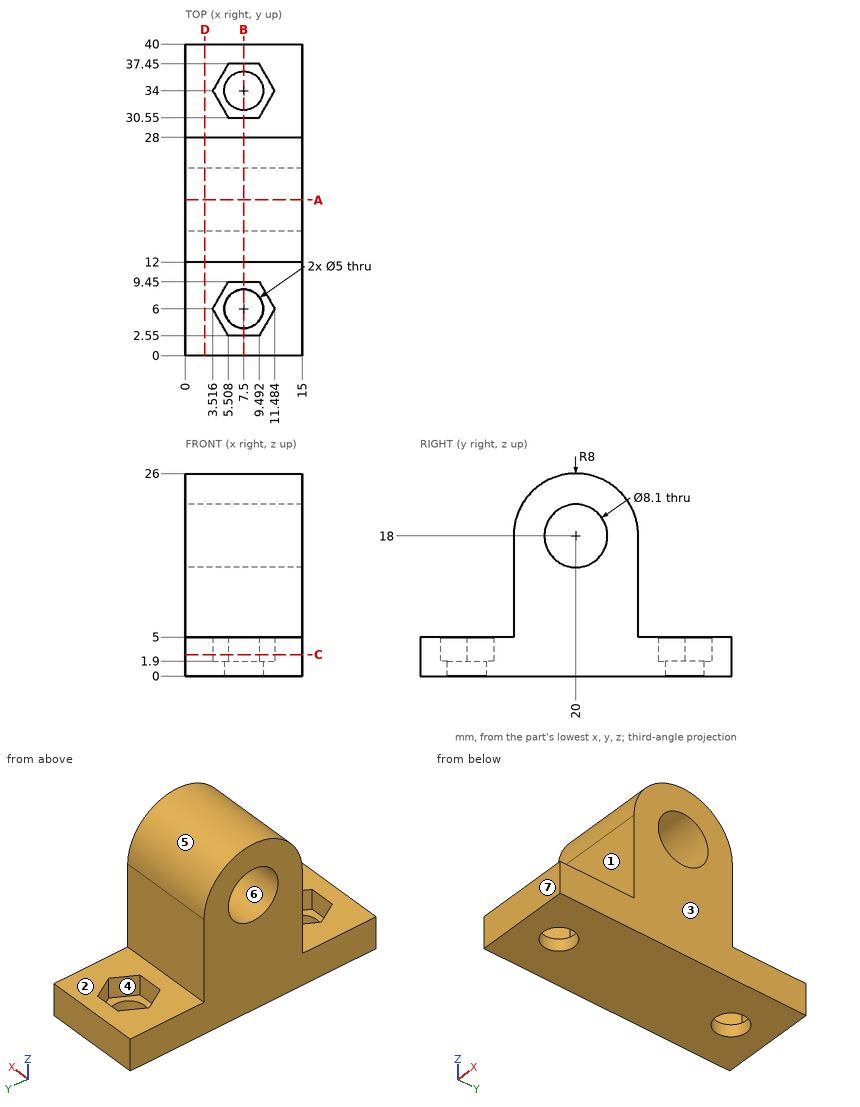
Geometry check sheet. Reference: drawing and pictorial views, mm from the part's lowest x, y, z. A direction names the side the tool comes from. Give positions to 0.01 mm unless a question says otherwise; leave off trailing zeros. Order: outer loops, then holes, each group sorted by start corner. A loop starts at its lowest first (then second) coordinate and runs counter-clockwise, first axis right, second up. Notation, with made-up numbers: (84, 18) -> (143, 18) arc R26 ccw to (143, 45) -> close; hole circle Ø2 at (9, 17.25). An arc over 180 degrees is marked (long way). Use CSV: the item, a comma, the result in double quotes. Start each with the question number.
1) Sectioned sample at A-A, the plane y = 20. Record the boundary of the cut face in (x, z).
2) Sectioned sample at C-C, the plane z = 2.75. Record the boundary of the cut face in (x, y).
3) Go/stop test with flat-tipped pins: P1, Ø2, axis at x = 7, y = 33.5, coming from the +Z side; P2, Ø5.5, axis at x = 7, y = 7, coming from the +Z side; P3, Ø4, axis at x = 11, z = 9, coming from the +Y side; P4, Ø4, axis at x = 4.5, z = 11.5, coming from the -Y side. Record where each tip stops, or that it passes through.
4) Sectioned sample at B-B, the plane x = 7.5. Record the boundary of the cut face in (y, z), plus the area to 3 significant figures.
5) Set-up check for the marked faces 1, 2 and 3: record each of +Z, -Z, +X, -X, +Y, -Y from which the full face is reachable in a straight line by a thin tool's end or side.
6) Material ranges on line 1 (X direction, y = 6, z = 0.8); line 2 (Z direction, x = 9.75, y = 20); line 3 (Z direction, x = 5, y = 18) (1 decimal), recorded low to high. Write a range as from..to.
7) Sectioned sample at D-D, the plane x = 2.5. Record the boundary of the cut face in (y, z), plus the area to 3 significant figures.
8) Mould release check, pull along Y, two halves, no side actions. Record for the marked faces 4, 5, 6 and 7: released by +Y, released by -Y, zero draft, split by the parting line, or undercut.
Recorded:
1,outline,"(0, 0) -> (15, 0) -> (15, 13.95) -> (0, 13.95) -> close; (0, 22.05) -> (15, 22.05) -> (15, 26) -> (0, 26) -> close"
2,outline,"(0, 0) -> (15, 0) -> (15, 40) -> (0, 40) -> close; hole (3.52, 6) -> (5.51, 2.55) -> (9.49, 2.55) -> (11.48, 6) -> (9.49, 9.45) -> (5.51, 9.45) -> close; hole (3.52, 34) -> (5.51, 30.55) -> (9.49, 30.55) -> (11.48, 34) -> (9.49, 37.45) -> (5.51, 37.45) -> close"
3,P1,"through"
3,P2,"z = 5"
3,P3,"y = 28"
3,P4,"y = 12"
4,outline,"(0, 0) -> (3.5, 0) -> (3.5, 1.9) -> (2.55, 1.9) -> (2.55, 5) -> (0, 5) -> close; (8.5, 0) -> (31.5, 0) -> (31.5, 1.9) -> (30.55, 1.9) -> (30.55, 5) -> (28, 5) -> (28, 18) arc R8 ccw to (12, 18) -> (12, 5) -> (9.45, 5) -> (9.45, 1.9) -> (8.5, 1.9) -> close; (36.5, 0) -> (40, 0) -> (40, 5) -> (37.45, 5) -> (37.45, 1.9) -> (36.5, 1.9) -> close; hole circle Ø8.1 at (20, 18)"
4,area,"395 mm2"
5,face 1,"+Z, +X, -X, -Y"
5,face 2,"+Z, +X, -X, +Y"
5,face 3,"+Z, -Z, +X, +Y, -Y"
6,line 1,"0..5, 10..15"
6,line 2,"0..13.95, 22.05..26"
6,line 3,"0..14.5, 21.5..25.7"
7,outline,"(0, 0) -> (40, 0) -> (40, 5) -> (28, 5) -> (28, 18) arc R8 ccw to (12, 18) -> (12, 5) -> (0, 5) -> close; hole circle Ø8.1 at (20, 18)"
7,area,"457 mm2"
8,face 4,"undercut"
8,face 5,"split by the parting line"
8,face 6,"undercut"
8,face 7,"released by -Y"
